```python
from build123d import *

# Parameters (mm, degrees)
SKETCH_R  = 2
PAD_DEPTH = 1.9


with BuildPart() as part:
    # Sketch → Pad (new body)
    with BuildSketch(Plane.XY):
        with BuildLine():
            ThreePointArc((3, -3), (4.5, 0), (3, 3))
            Line((3, 3), (3, 5.3))
            Line((-3, 5.3), (3, 5.3))
            Line((-3, 3), (-3, 5.3))
            ThreePointArc((-3, 3), (-4.5, 0), (-3, -3))
            Line((-3, -3), (-3, -5.3))
            Line((3, -5.3), (-3, -5.3))
            Line((3, -3), (3, -5.3))
        make_face()
        Circle(SKETCH_R, mode=Mode.SUBTRACT)
    extrude(amount=PAD_DEPTH)


solid = part.part
```
Model file for the job. Use its own axes, mm. A direction names the side the tool comes from. Give positions to 0.01 mm unless a question says otherwise; leave off trailing zeros. Order: outer loops, then holes, each group sorted by start corner. A loop starts at its lowest first (then second) coordinate and runs counter-clockwise, first axis right, second up.
1) 3-axis set-ups, long thin cutter, end or side, ignore diameter. For faces 1 (the cylindrical face through (-4.5, 0, 0.9)), 2 (the flat face through (2, 1, 1.9)), 3 (the flat face through (3, -4, 1)), 4 (the flat face through (-3, 4, 1)), 5 (the flat face through (3, 4, 1)): which of +Z, -Z, +X, -X, +Y, -Y reach the whole face in a straight line?
2) Mould opens along Y. For faces 6 (the flat face through (0, -5.3, 1)), 7 (the cylindrical face through (0, -2, 1)), 8 (the flat face through (-3, -4, 1)), 9 (the cylindrical face through (4.5, 0, 0.9)) say: +Y half, -Y half, draft (parallel to the pull), parting line (faces both ways), or undercut.
3) Saw through at C-C, the plane z = 1.5. Write the cut outline in (x, y), then the cut area to 3 significant figures.
4) Pin check, flat tips, straight feed: pin 1 (0.6 mm diameter, centred on y = -4, z = 1, fed in from +X); pin 2 (3 mm diameter, centred on x = -1, y = -3, fed in from -Z); pin 3 (1 mm diameter, centred on y = -4, z = 0.5, fed in from -X). Stop position of each tip, or through.
5) Wall check: probe 1 along Y at (x, z) = (0, 0.75); probe 2 along X at (y, z) = (-1.75, 1.5); probe 3 along X at (y, z) = (0.5, 0.8). Give the ranges that are in metal, low to high.
6) Saw through at A-A, the plane y = 0. Write the cut outline in (x, z).
7) Saw through at B-B, the plane x = 0. Write the cut outline in (y, z).
8) Saw through at D-D, the plane y = 2.5. Write the cut outline in (x, z).
Computed:
1. face 1: +Z, -Z, -X
1. face 2: +Z, +X, -X, +Y, -Y
1. face 3: +Z, -Z, +X, -Y
1. face 4: +Z, -Z, -X, +Y
1. face 5: +Z, -Z, +X, +Y
2. face 6: -Y half
2. face 7: undercut
2. face 8: draft
2. face 9: parting line
3. outline: (-3, -5.3) - (3, -5.3) - (3, -3) arc R3.75 ccw to (3, 3) - (3, 5.3) - (-3, 5.3) - (-3, 3) arc R3.75 ccw to (-3, -3) - close; hole circle Ø4 at (0, 0)
3. area: 63.6 mm2
4. pin 1: stops at x = 3
4. pin 2: stops at z = 0
4. pin 3: stops at x = -3
5. probe 1: y = -5.3 to -2, 2 to 5.3
5. probe 2: x = -4.07 to -0.97, 0.97 to 4.07
5. probe 3: x = -4.47 to -1.94, 1.94 to 4.47
6. outline: (-4.5, 0) - (-2, 0) - (-2, 1.9) - (-4.5, 1.9) - close; (2, 0) - (4.5, 0) - (4.5, 1.9) - (2, 1.9) - close
7. outline: (-5.3, 0) - (-2, 0) - (-2, 1.9) - (-5.3, 1.9) - close; (2, 0) - (5.3, 0) - (5.3, 1.9) - (2, 1.9) - close
8. outline: (-3.55, 0) - (3.55, 0) - (3.55, 1.9) - (-3.55, 1.9) - close
